from build123d import *

# Parameters (mm, degrees)
ESQUISSE2_W             = 251
ESQUISSE2_H             = 25
ESQUISSE2_R             = 4.05
ESQUISSE2_R_2           = 1
ESQUISSE2_R_3           = 1.5
ESQUISSE2_W_2           = 5
ESQUISSE2_H_2           = 5
BOSS_EXTRU_1_DEPTH      = 2
CONG_1_R                = 5
ESQUISSE3_R             = 1.5
ESQUISSE3_W             = 5
ESQUISSE3_H             = 5
ENL_V_MAT_EXTRU_1_DEPTH = 10


with BuildPart() as part:
    # Esquisse2 → Boss.-Extru.1 (new body)
    with BuildSketch(Plane(origin=(0, 0, 0), x_dir=(-1, 0, 0), z_dir=(0, 0, -1))):
        with Locations((-125.5, 0)):
            Rectangle(ESQUISSE2_W, ESQUISSE2_H)
        with Locations((-11, 0)):
            Circle(ESQUISSE2_R, mode=Mode.SUBTRACT)
        with Locations((-4, 0)):
            Circle(ESQUISSE2_R_2, mode=Mode.SUBTRACT)
        with Locations((-4.937822174, -3.5)):
            Circle(ESQUISSE2_R_2, mode=Mode.SUBTRACT)
        with Locations((-7.5, -6.062177826)):
            Circle(ESQUISSE2_R_2, mode=Mode.SUBTRACT)
        with Locations((-11, -7)):
            Circle(ESQUISSE2_R_2, mode=Mode.SUBTRACT)
        with Locations((-14.5, -6.062177826)):
            Circle(ESQUISSE2_R_2, mode=Mode.SUBTRACT)
        with Locations((-17.062177826, -3.5)):
            Circle(ESQUISSE2_R_2, mode=Mode.SUBTRACT)
        with Locations((-18, 0)):
            Circle(ESQUISSE2_R_2, mode=Mode.SUBTRACT)
        with Locations((-17.062177826, 3.5)):
            Circle(ESQUISSE2_R_2, mode=Mode.SUBTRACT)
        with Locations((-14.5, 6.062177826)):
            Circle(ESQUISSE2_R_2, mode=Mode.SUBTRACT)
        with Locations((-11, 7)):
            Circle(ESQUISSE2_R_2, mode=Mode.SUBTRACT)
        with Locations((-7.5, 6.062177826)):
            Circle(ESQUISSE2_R_2, mode=Mode.SUBTRACT)
        with Locations((-4.937822174, 3.5)):
            Circle(ESQUISSE2_R_2, mode=Mode.SUBTRACT)
        with Locations((-243.5, 0)):
            Circle(ESQUISSE2_R_3, mode=Mode.SUBTRACT)
        with BuildLine():
            Line((-26, -2.1), (-41, -2.1))
            ThreePointArc((-41, -2.1), (-43.1, 0), (-41, 2.1))
            Line((-41, 2.1), (-26, 2.1))
            ThreePointArc((-26, 2.1), (-23.9, 0), (-26, -2.1))
        make_face(mode=Mode.SUBTRACT)
        with Locations((-243.5, -7.5)):
            Rectangle(ESQUISSE2_W_2, ESQUISSE2_H_2, mode=Mode.SUBTRACT)
        with Locations((-243.5, 7.5)):
            Rectangle(ESQUISSE2_W_2, ESQUISSE2_H_2, mode=Mode.SUBTRACT)
    extrude(amount=-BOSS_EXTRU_1_DEPTH)

    # Congé1
    cong_1_edges = [part.edges().sort_by_distance(p)[0] for p in [
        (251, 12.5, 1),
        (0, 12.5, 1),
        (0, -12.5, 1),
        (251, -12.5, 1),
    ]]
    fillet(cong_1_edges, radius=CONG_1_R)

    # Esquisse3 → Enlèv. mat.-Extru.1 (cut)
    with BuildSketch(Plane(origin=(0, 0, 0), x_dir=(-1, 0, 0), z_dir=(0, 0, -1))):
        with Locations((-243.5, 0)):
            Circle(ESQUISSE3_R)
        with Locations((-213.5, 0)):
            Circle(ESQUISSE3_R)
        with Locations((-243.5, -7.5)):
            Rectangle(ESQUISSE3_W, ESQUISSE3_H)
        with Locations((-243.5, 7.5)):
            Rectangle(ESQUISSE3_W, ESQUISSE3_H)
        with Locations((-213.5, -7.5)):
            Rectangle(ESQUISSE3_W, ESQUISSE3_H)
        with Locations((-213.5, 7.5)):
            Rectangle(ESQUISSE3_W, ESQUISSE3_H)
        with BuildLine():
            Line((-230, -7.5), (-230, 7.5))
            ThreePointArc((-230, 7.5), (-228.5, 9), (-227, 7.5))
            Line((-227, 7.5), (-227, -7.5))
            ThreePointArc((-227, -7.5), (-228.5, -9), (-230, -7.5))
        make_face()
    extrude(amount=-ENL_V_MAT_EXTRU_1_DEPTH, mode=Mode.SUBTRACT)


solid = part.part
Verification items for the finished model (mm, model axes). Give positions to 0.01 mm unless a question says otherwise; leave off trailing zeros. Answer as CSV lines item,"result". Start each with the question number.
1. Draft check along Y on faces 1 (the face through (249.57, -11, 1.01)), 2 (the face through (1.5, 11.07, 1.01)), 3 (the face through (11.878, -3.954, 0.986)). Enter one of: pulls with the +Y half, pulls with the -Y half, needs draft (parallel to the pull), parting line crosses it, or undercut.
2. Sectioned sample at A-A (z = 1.05). Count the separate pieces of the cut face and the enclosed holes in it, then the cut area to 3 significant figures.
3. Thickness scan on line 1 (Y direction, x = 11, z = 0.6); line 2 (X direction, y = -9.5, z = 1.45); line 3 (X direction, y = -9.25, z = 0.6). Record the ranges inside material, lowest first.
4. Depth check by flat-ended pin: pin 1 (0.6 mm diameter, centred on y = -8.5, z = 1.5, fed in from +X); pin 2 (1.8 mm diameter, centred on x = 7.5, y = -6.06, fed in from +Z). Enter the tip coordinate at first touch or a pass-through.
Derived:
1,face 1,"pulls with the -Y half"
1,face 2,"pulls with the +Y half"
1,face 3,"undercut"
2,separate pieces,"1"
2,enclosed holes,"21"
2,area,"5,920 mm²"
3,line 1,"-12.5 to -8, -6 to -4.05, 4.05 to 6, 8 to 12.5"
3,line 2,"0.42 to 211, 216 to 241, 246 to 250.58"
3,line 3,"0.32 to 211, 216 to 241, 246 to 250.68"
4,pin 1,"x = 250.95"
4,pin 2,"through"
